Autodesk Inventor part; units mm, degrees
ref_plane "YZ Plane" through (0, 0, 0) normal (1, 0, 0) x (0, 1, 0)
ref_plane "XZ Plane" through (0, 0, 0) normal (0, 1, 0) x (-1, 0, 0)
ref_plane "XY Plane" through (0, 0, 0) normal (0, 0, 1) x (1, 0, 0)
sketch "Sketch1" plane through (0, 0, 0) normal (1, 0, 0) x (0, 1, 0)
  line L0 (6.9282, 0) -> (3.4641, -6)
  line L1 (3.4641, -6) -> (-3.4641, -6)
  line L2 (-3.4641, -6) -> (-6.9282, 0)
  line L3 (-6.9282, 0) -> (-3.4641, 6)
  line L4 (-3.4641, 6) -> (3.4641, 6)
  line L5 (3.4641, 6) -> (6.9282, 0)
  circle A0 centre (0, 0) radius 4.15
  dimension "d0" = 12
  dimension "d1" = 8.3
extrude "Extrusion1" add sketch "Sketch1" along normal mid plane 2
thread "Thread1"
properties part number "Porca do Plug P10"
Build history of the part. All positions in model axes, mm. Round coordinates to 2 decimals unless told otherwise and drop trailing zeros. Write each loop counter-clockwise with the first axis right and the second up, starting at its lowest first coordinate (ties: lowest second). Pieces come first, ordered by that corner, then holes. Notation, with made-up numbers: (46.5, 83.25) - (52.5, 83.25) arc R11 ccw to (52.5, 95.25) - close; hole circle Ø5 at (-17, 42). An arc over 180 degrees is marked (long way). Answer as CSV lines item,"result".
Q1. Cut at B-B (x = 0.1). Write the cut outline in (y, z).
Report:
outline,"(-6.93, 0) - (-3.46, -6) - (3.46, -6) - (6.93, 0) - (3.46, 6) - (-3.46, 6) - close; hole circle Ø8.3 at (0, 0)"
Q2. Cut at C-C (z = -3). Write the cut outline in (x, y), and give its area (3 significant figures).
Report:
outline,"(-1, -5.2) - (1, -5.2) - (1, -2.87) - (-1, -2.87) - close; (-1, 2.87) - (1, 2.87) - (1, 5.2) - (-1, 5.2) - close"
area,"9.31 mm^2"
Q3. Pull direction Y, two halves, no side cores. Call faces 1 (the cylindrical face through (-0.01, -0.9, 4.05)), 2 (the flat face through (-0.01, -5.22, 2.96)), 3 (the flat face through (-0.01, 5.22, -2.96)): +Y half, -Y half, draft (parallel to the pull), parting line (faces both ways), or undercut.
Report:
face 1,"undercut"
face 2,"-Y half"
face 3,"+Y half"
Q4. Cut at A-A (y = 0). Write the cut outline in (x, z), and give its area (3 significant figures).
Report:
outline,"(-1, -6) - (1, -6) - (1, -4.15) - (-1, -4.15) - close; (-1, 4.15) - (1, 4.15) - (1, 6) - (-1, 6) - close"
area,"7.40 mm^2"
Q5. Cut at D-D (z = -4.75). Write the cut outline in (x, y).
Report:
outline,"(-1, -4.19) - (1, -4.19) - (1, 4.19) - (-1, 4.19) - close"
Q6. Drill centre lines: probe 1 along Z at (x, y) = (0.2, 0); probe 2 along Z at (x, y) = (-0.35, -3.5); probe 3 along Y at (x, z) = (-0.2, -2.75). Where is each one in solid material? Low to high. Write a range as [from, to].
Report:
probe 1,"z = [-6, -4.15], [4.15, 6]"
probe 2,"z = [-5.94, -2.23], [2.23, 5.94]"
probe 3,"y = [-5.34, -3.11], [3.11, 5.34]"
Q7. Drop a flat-ended pin along its axis: pin 1 (3 mm diameter, centred on y = -4, z = -0.5, fed in from -X). Give the stop position or say it passes through.
Report:
pin 1,"stops at x = -1"
